Verification items for the finished model (mm, model axes). Face numbers are marked on the shaded views. A direction names the side the tool comes from. Give positions to 0.01 mm unless a question says otherwise; leave off trailing zeros. Order: outer loops, then holes, each group sorted by start corner. A loop starts at its lowest first (then second) coordinate and runs counter-clockwise, first axis right, second up. Notation, with made-up numbers: M 45,41 L 103,41 A19 ccw 103,74 Z; hole C 71,68.5 d5. An arc over 180 degrees is marked long. Answer as a JSON object with one key per item and string values.
```python
from build123d import *

# Parameters (mm, degrees)
F0_R      = 98
F1_DEPTH  = 900
F2_R      = 98
F2_R_2    = 50
F3_DEPTH  = 200
F4_SIZE   = 40
F5_R      = 5
F8_DEPTH  = 50
F9_R      = 6.75
F9_R_2    = 10
F10_DEPTH = 10.001


# Not quite as in the source:
# - a pattern or mirror of a feature is missing from the dataset's text; its kind, count and spacing are read off the source's solid


with BuildPart() as f1:
    # F0 (on Top) → F1 (new body, symmetric)
    with BuildSketch(Plane.XY):
        Circle(F0_R)
    extrude(amount=F1_DEPTH, both=True)

    # F2 (on face) → F3 (cut)
    with BuildSketch(Plane(origin=(0, 0, -900), x_dir=(1, 0, 0), z_dir=(0, 0, -1))):
        Circle(F2_R)
        Circle(F2_R_2, mode=Mode.SUBTRACT)
    extrude(amount=-F3_DEPTH, mode=Mode.SUBTRACT)

    # F4
    f4_edges = [f1.edges().sort_by_distance(p)[0] for p in [
        (-50, 0, -700),
    ]]
    chamfer(f4_edges, length=F4_SIZE)

    # F5
    f5_edges = [f1.edges().sort_by_distance(p)[0] for p in [
        (-50, 0, -900),
        (-98, 0, 900),
    ]]
    fillet(f5_edges, radius=F5_R)

    # F7 (on offset) → F8 (join)
    with BuildSketch(Plane(origin=(0, 0, -680), x_dir=(1, 0, 0), z_dir=(0, 0, -1))):
        Polygon((76.2233031652, -72.2150126676), (65.2159465136, -73.14971169), (132.6794919243, -190), (-132.6794919243, -190), (-65.2159465136, -73.14971169), (-76.2233031652, -72.2150126676), (-144.2264973081, -190), (-200, -190), (-200, -200), (-150, -200), (150, -200), (200, -200), (200, -190), (144.2264973081, -190), align=None)
        with BuildLine():
            ThreePointArc((-65.2159465136, -73.14971169), (0, 98), (65.2159465136, -73.14971169))
            Line((65.2159465136, -73.14971169), (76.2233031652, -72.2150126676))
            ThreePointArc((76.2233031652, -72.2150126676), (0, 105), (-76.2233031652, -72.2150126676))
            Line((-76.2233031652, -72.2150126676), (-65.2159465136, -73.14971169))
        make_face()
    f8 = extrude(amount=-F8_DEPTH)

    # F8_copies: F8 across plane
    add(f8.mirror(Plane.XY.offset(70)))

    # F9 (on face) → F10 (cut, through all)
    with BuildSketch(Plane.XZ.offset(-190)):
        with Locations((-172.1132486541, -655)):
            Circle(F9_R)
        with Locations((176.858574152, -655)):
            Circle(F9_R_2)
    f10 = extrude(amount=-F10_DEPTH, mode=Mode.SUBTRACT)

    # F10_copies: F10 across plane
    add(f10.mirror(Plane.XY.offset(70)), mode=Mode.SUBTRACT)


solid = f1.part
```
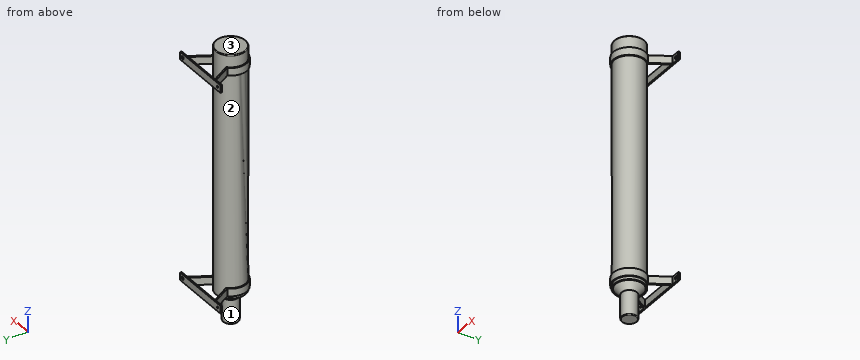
Q1. Tool access check on the marked faces 1, 2 and 3. Record the directions out of +Z, -Z, +X, -X, +Y, -Y that give a thin tool (end or side, any length) a straight path to the whole face; none if there is none.
Resolved:
{"face 1": "-Z", "face 2": "none", "face 3": "+Z, +X, -X, +Y, -Y"}
Q2. Material ranges on L1, parallel to X at y = 194, z = -655; L2, parallel to Y at x = -2, z = 725.5; L3, parallel to Y at x = -28, z = -197, recorded low to high.
Resolved:
{"L1": "x = -200 to -178.86, -165.36 to 166.86, 186.86 to 200", "L2": "y = -97.98 to 97.98", "L3": "y = -93.91 to 93.91"}
Q3. Gauge pin test, flat ends, axial feed: pin 1 Ø12 at (x, z) = (-57.5, 164.5) entering from +Y; pin 2 Ø1.5 at (x, y) = (-103.5, 135) entering from -Z; pin 3 Ø15 at (x, z) = (-170, -643.5) entering from -Y; pin 4 Ø12 at (x, z) = (-172.11, -655) entering from -Y. Record the tip position at first contact, or that the pin passes through.
Resolved:
{"pin 1": "stops at y = 83.38", "pin 2": "stops at z = -680", "pin 3": "stops at y = 190", "pin 4": "passes through"}
Q4. Section check A-A on x = 0. Count the separate pieces of the cut face and the enclosed holes in it, then the cut area to 3 significant figures.
Resolved:
{"separate pieces": "3", "enclosed holes": "0", "area": "337,000 mm²"}
Q5. Section check C-C on z = 529. Record the cut outline in (x, y).
Resolved:
{"outline": "C 0,0 d196"}
